Build history of the part. All positions in model axes, mm. A direction names the side the tool comes from. Round coordinates to 2 decimals unless told otherwise and drop trailing zeros. Write each loop counter-clockwise with the first axis right and the second up, starting at its lowest first coordinate (ties: lowest second). Pieces come first, ordered by that corner, then holes. Notation, with made-up numbers: M 27.5,-19 L 45.5,-19 A35 cw 45.5,19 Z; hole C 75,64.25 d8. An arc over 180 degrees is marked long. Write item = value, one per line.
from build123d import *

# Parameters (mm, degrees)
F0_W     = 152.4
F0_H     = 101.6
F1_DEPTH = 152.4
F3_D     = 279.4
F0_W_2   = 50.8
F4_DEPTH = 12.7


with BuildPart() as f1:
    # F0 (on Top) → F1 (new body)
    with BuildSketch(Plane.XY):
        with Locations((-127, 50.8)):
            Rectangle(F0_W, F0_H)
    extrude(amount=F1_DEPTH)

    # F3 (through all)
    with Locations(Plane.XZ):
        with Locations((-50.8, 152.4)):
            Hole(F3_D / 2)

    # F0 (on Top) → F4 (join)
    with BuildSketch(Plane.XY):
        with Locations((-25.4, 50.8)):
            Rectangle(F0_W_2, F0_H)
    extrude(amount=F4_DEPTH)

    # F5: F1 across plane


with BuildPart() as f1_1:
    add(f1.part)
    add(f1.part.mirror(Plane.XZ))

    # F6: F1 across plane


with BuildPart() as f1_2:
    add(f1_1.part)
    add(f1_1.part.mirror(Plane.YZ))


solid = f1_2.part
1. Band-saw the part on D-D (z = 135). List the corners of the cut face in (x, y).
Responses:
outline = M -203.2,-101.6 L -189.41,-101.6 L -189.41,101.6 L -203.2,101.6 Z; M 189.41,-101.6 L 203.2,-101.6 L 203.2,101.6 L 189.41,101.6 Z
2. Tool access for faces 1 (the face through (1, -1, 12.7)), 2 (the face through (-197, 1, 152.4)): list every direction of +Z, -Z, +X, -X, +Y, -Y with a clear straight run to the whole face (end or side of a thin tool).
Responses:
face_1 = +Z, +Y, -Y
face_2 = +Z, +X, -X, +Y, -Y
3. Probe probe 1 along X at (y, z) = (-54, 29.5); probe 2 along X at (y, z) = (-30.5, 108); probe 3 along Z at (x, y) = (-3, 5.5). List the from-to ranges inside material, lowest first.
Responses:
probe_1 = -203.2 to -117.22, 117.22 to 203.2
probe_2 = -203.2 to -183.26, 183.26 to 203.2
probe_3 = 0 to 12.7
4. Band-saw the part on A-A (z = 65). List the corners of the cut face in (x, y), plus the area to 3 significant figures.
Responses:
outline = M -203.2,-101.6 L -159.78,-101.6 L -159.78,101.6 L -203.2,101.6 Z; M 159.78,-101.6 L 203.2,-101.6 L 203.2,101.6 L 159.78,101.6 Z
area = 17,600 mm²
5. Flat gauge pins, fed straight in: pin 1 (1.5 mm diameter, centred on x = 22, y = 2, fed in from +Z); pin 2 (8 mm diameter, centred on x = 51, y = -26, fed in from +Z); pin 3 (5 mm diameter, centred on x = 159.5, y = 21, fed in from +Z). Where does each tip first touch, or does it go through?
Responses:
pin_1 = 12.7
pin_2 = 12.76
pin_3 = 67.84
6. Mould opens along X. For faces 3 (the face through (3, 1, 0)), 4 (the face through (148.491, -1.422, 52.537)), 5 (the face through (203.2, -1, 75)) say: pulls with the +X half, pulls with the -X half, needs draft (parallel to the pull), parting line crosses it, or undercut.
Responses:
face_3 = needs draft
face_4 = undercut
face_5 = pulls with the +X half
7. Band-saw the part on C-C (x = -4). List the corners of the cut face in (y, z), plus the area to 3 significant figures.
Responses:
outline = M -101.6,0 L 101.6,0 L 101.6,12.7 L -101.6,12.7 Z
area = 2,580 mm²
8. Band-saw the part on B-B (y = -9.5). List the corners of the cut face in (x, z), plus the area to 3 significant figures.
Responses:
outline = M -203.2,0 L 203.2,0 L 203.2,152.4 L 190.5,152.4 A139.7 cw 50.8,12.7 L -50.8,12.7 A139.7 cw -190.5,152.4 L -203.2,152.4 Z
area = 17,100 mm²
